from build123d import *

# Parameters (mm, degrees)
SKETCH1_W           = 497
SKETCH1_H           = 176.5
BOSS_EXTRUDE1_DEPTH = 18
SKETCH4_R           = 2.5
CUT_EXTRUDE3_DEPTH  = 18
SKETCH5_R           = 10
CUT_EXTRUDE4_DEPTH  = 18


with BuildPart() as part:
    # Sketch1 → Boss-Extrude1 (new body)
    with BuildSketch(Plane.XY):
        with Locations((0, -123.25)):
            Rectangle(SKETCH1_W, SKETCH1_H)
    extrude(amount=BOSS_EXTRUDE1_DEPTH)

    # Sketch4 → Cut-Extrude3 (cut)
    with BuildSketch(Plane.XY.offset(18)):
        with Locations((64, -123.25)):
            Circle(SKETCH4_R)
        with Locations(Location((-64, -123.25, 0), (0, 0, 180))):
            Circle(SKETCH4_R)
    extrude(amount=-CUT_EXTRUDE3_DEPTH, mode=Mode.SUBTRACT)

    # Sketch5 → Cut-Extrude4 (cut)
    with BuildSketch(Plane.XY.offset(18)):
        with Locations((148.5, -70)):
            Circle(SKETCH5_R)
    extrude(amount=-CUT_EXTRUDE4_DEPTH, mode=Mode.SUBTRACT)


solid = part.part
Work out the finished part from the listing and answer in its coordinate system (mm). Coordinates: 2 decimals unless noted, no trailing zeros. Order: outer loops, then holes, each group sorted by start corner. A loop starts at its lowest first (then second) coordinate and runs counter-clockwise, first axis right, second up. Notation, with made-up numbers: (-13, 3) - (-8, 3) arc R15 ccw to (-8, 24) - close; hole circle Ø8 at (-9.5, -11). An arc over 180 degrees is marked (long way). Put each result on its own line as item: value. Start each with the question number.
1) Find section A-A (x = 148.5). Give the vertices of the cut face in (y, z).
2) Find section B-B (y = -75). Give the vertices of the cut face in (x, z), plus the area to 3 significant figures.
3) Find the intervals of material crossed by line 1 (Y direction, x = -64, z = 10); line 2 (Y direction, x = 148.5, z = 6); line 3 (X direction, y = -74, z = 13.75), in increasing order. Write a range as from..to.
4) For a pull along X with two mould halves and no side action, classify faces 1 (the flat face through (248.5, -124, 9)), 2 (the cylindrical face through (157.737, -73.83, 9.126)), 3 (the flat face through (-3, -122, 0)) as released by +X, released by -X, zero draft, split by the parting line, or undercut.
5) Flat-ended cylindrical pins translate along their axes: pin 1 (6 mm diameter, centred on x = -64, y = -123.25, fed in from +Z); pin 2 (12 mm diameter, centred on x = 148.5, y = -70, fed in from +Z). Find the tip coordinate at first contact, or state that the pin passes through.
Results list:
1. outline: (-211.5, 0) - (-80, 0) - (-80, 18) - (-211.5, 18) - close; (-60, 0) - (-35, 0) - (-35, 18) - (-60, 18) - close
2. outline: (-248.5, 0) - (139.84, 0) - (139.84, 18) - (-248.5, 18) - close; (157.16, 0) - (248.5, 0) - (248.5, 18) - (157.16, 18) - close
2. area: 8,630 mm^2
3. line 1: y = -211.5..-125.75, -120.75..-35
3. line 2: y = -211.5..-80, -60..-35
3. line 3: x = -248.5..139.33, 157.67..248.5
4. face 1: released by +X
4. face 2: undercut
4. face 3: zero draft
5. pin 1: stops at z = 18
5. pin 2: passes through
